Geometry check sheet. Reference: the model listing, model coordinates, mm. A direction names the side the tool comes from. Give positions to 0.01 mm unless a question says otherwise; leave off trailing zeros. Order: outer loops, then holes, each group sorted by start corner. A loop starts at its lowest first (then second) coordinate and runs counter-clockwise, first axis right, second up. Notation, with made-up numbers: M 30.5,32.5 L 79.5,32.5 A13 cw 79.5,38.5 Z; hole C -17.75,86 d5. An arc over 180 degrees is marked long. Put each result on its own line as item: value. Start each with the question number.
Q1. Access from +Z, -Z, +X, -X, +Y, -Y to the whole of each face (thin tool, end or side, straight path). Record for faces 1 (the flat face through (-50, -25, -1)), 2 (the flat face through (-1, -25, 100)), 3 (the flat face through (45.5, -25, 1)), 4 (the flat face through (-1, -25, -100)).
Q2. Section check A-A on z = -73. Record the cut outline in (x, y).
Q3. Section check B-B on x = -27. Record the cut outline in (y, z).
Q4. Mould release check, pull along Y, two halves, no side actions. Record for faces 5 (the flat face through (50, -25, -1)), 6 (the flat face through (-3, 10, -4)), 7 (the flat face through (25, -36, 1)): +Y half, -Y half, draft (parallel to the pull), parting line (faces both ways), or undercut.
Q5. Material ranges on L1, parallel to X at y = -17, z = 74.5; L2, parallel to Y at x = 168, z = -230; L3, parallel to X at y = -45.5, z = 96, recorded low to high.
Q6. Go/stop test with flat-tipped pins: pin 1 (17.5 mm diameter, centred on y = -29.5, z = 18, fed in from -X); pin 2 (17.5 mm diameter, centred on y = -26, z = -36, fed in from +X); pin 3 (2 mm diameter, centred on x = -166.5, z = 122, fed in from -Y). Record where each tip stops, or that it passes through.
Q7. Section check C-C on z = 172.5. Record the cut outline in (x, y), then the cut area to 3 significant figures.
Q8. Section check D-D on x = 80. Record the cut outline in (y, z), then the cut area to 3 significant figures.
```python
from build123d import *

# Parameters (mm, degrees)
SKETCH1_W           = 500
SKETCH1_H           = 500
BOSS_EXTRUDE1_DEPTH = 10
SKETCH2_W           = 100
SKETCH2_H           = 200
BOSS_EXTRUDE2_DEPTH = 50
CUT_EXTRUDE1_REACH  = 435.013
SKETCH3_W           = 41
SKETCH3_H           = 22


with BuildPart() as part:
    # Sketch1 → Boss-Extrude1 (new body)
    with BuildSketch(Plane(origin=(0, 0, 0), x_dir=(1, 0, 0), z_dir=(0, 1, 0))):
        Rectangle(SKETCH1_W, SKETCH1_H)
    extrude(amount=BOSS_EXTRUDE1_DEPTH)

    # Sketch2 → Boss-Extrude2 (add)
    with BuildSketch(Plane.XZ):
        Rectangle(SKETCH2_W, SKETCH2_H)
    extrude(amount=BOSS_EXTRUDE2_DEPTH)

    # Sketch3 → Cut-Extrude1 (cut, up to next)
    with BuildSketch(Plane.XY.offset(100), mode=Mode.PRIVATE) as cut_extrude1_sk1:
        with Locations((-25, -25)):
            Rectangle(SKETCH3_W, SKETCH3_H)
    cut_extrude1_tool1 = extrude(cut_extrude1_sk1.sketch, amount=-CUT_EXTRUDE1_REACH, mode=Mode.PRIVATE) & part.part
    # Sketch3 → Cut-Extrude1 (cut, up to next)
    with BuildSketch(Plane.XY.offset(100), mode=Mode.PRIVATE) as cut_extrude1_sk2:
        with Locations((25, -25)):
            Rectangle(SKETCH3_W, SKETCH3_H)
    cut_extrude1_tool2 = extrude(cut_extrude1_sk2.sketch, amount=-CUT_EXTRUDE1_REACH, mode=Mode.PRIVATE) & part.part
    add(cut_extrude1_tool1.solids().sort_by_distance((-25, -25, 100))[0], mode=Mode.SUBTRACT)
    add(cut_extrude1_tool2.solids().sort_by_distance((25, -25, 100))[0], mode=Mode.SUBTRACT)


solid = part.part
```
Results found:
1. face 1: +Z, -Z, -X, -Y
1. face 2: +Z, +X, -X, -Y
1. face 3: +Z, -Z
1. face 4: -Z, +X, -X, -Y
2. outline: M -250,0 L -50,0 L -50,-50 L 50,-50 L 50,0 L 250,0 L 250,10 L -250,10 Z; hole M -45.5,-36 L -4.5,-36 L -4.5,-14 L -45.5,-14 Z; hole M 4.5,-36 L 45.5,-36 L 45.5,-14 L 4.5,-14 Z
3. outline: M -50,-100 L -36,-100 L -36,100 L -50,100 Z; M -14,-100 L 0,-100 L 0,-250 L 10,-250 L 10,250 L 0,250 L 0,100 L -14,100 Z
4. face 5: draft
4. face 6: +Y half
4. face 7: undercut
5. L1: x = -50 to -45.5, -4.5 to 4.5, 45.5 to 50
5. L2: y = 0 to 10
5. L3: x = -50 to 50
6. pin 1: stops at x = -50
6. pin 2: stops at x = 50
6. pin 3: stops at y = 0
7. outline: M -250,0 L 250,0 L 250,10 L -250,10 Z
7. area: 5,000 mm^2
8. outline: M 0,-250 L 10,-250 L 10,250 L 0,250 Z
8. area: 5,000 mm^2
